Print and shaded views of the part. All mm, measured from the part's lowest x, y and z. A direction names the side the tool comes from. Coordinates: 2 decimals unless noted, no trailing zeros. Order: outer loops, then holes, each group sorted by start corner. A loop starts at its lowest first (then second) coordinate and runs counter-clockwise, first axis right, second up.
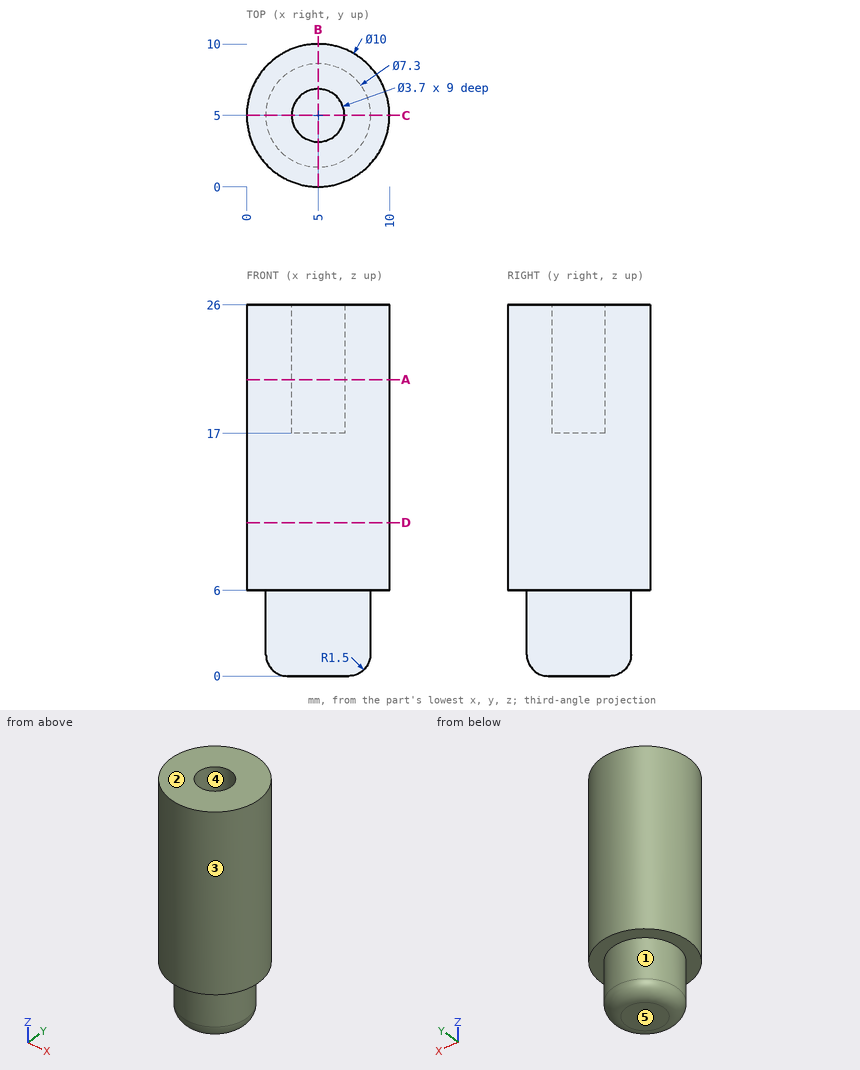
Q1. Cut at B-B, the plane x = 5. List the corners of the cut face in (y, z).
Established:
outline: (0, 6) - (1.35, 6) - (1.35, 1.5) arc R1.5 ccw to (2.85, 0) - (7.15, 0) arc R1.5 ccw to (8.65, 1.5) - (8.65, 6) - (10, 6) - (10, 26) - (6.85, 26) - (6.85, 17) - (3.15, 17) - (3.15, 26) - (0, 26) - close
Q2. Mould opens along X. For the marked faces 3, 4 and 5 say: pulls with the +X half, pulls with the -X half, needs draft (parallel to the pull), parting line crosses it, or undercut.
Established:
face 3: parting line crosses it
face 4: undercut
face 5: needs draft
Q3. Cut at A-A, the plane z = 20.75. List the corners of the cut face in (x, y), plus the area to 3 significant figures.
Established:
outline: circle Ø10 at (5, 5); hole circle Ø3.7 at (5, 5)
area: 67.8 mm2
Q4. Drop flat-ended pins along their axis: P1, Ø5, axis at x = 5, y = 5, coming from the +Z side; P2, Ø1, axis at x = 1.5, z = 10, coming from the -Y side; P3, Ø6, axis at x = 1.5, z = 3.5, coming from the -Y side; P4, Ø2, axis at x = 2.5, y = 7.5, coming from the -Z side. Give the stop position or say it passes through.
Established:
P1: stops at z = 26
P2: stops at y = 1
P3: stops at y = 0.35
P4: stops at z = 0.05
Q5. Cut at D-D, the plane z = 10.75. List the corners of the cut face in (x, y), plus the area to 3 significant figures.
Established:
outline: circle Ø10 at (5, 5)
area: 78.5 mm2
Q6. Probe line 1 (Y direction, x = 5, z = 21); line 2 (Z direction, x = 2.75, y = 8); line 3 (Z direction, x = 5.5, y = 6.75). List the from-to ranges inside material, lowest first.
Established:
line 1: y = 0 to 3.15, 6.85 to 10
line 2: z = 6 to 26
line 3: z = 0 to 17
Q7. Which spindle directions (+Z, -Z, +X, -X, +Y, -Y) get a long thin tool onto all of the face, cutting with end or side? Do the marked faces 1 and 2. Say none if no direction does.
Established:
face 1: -Z
face 2: +Z, +X, -X, +Y, -Y
